```python
from build123d import *

# Parameters (mm, degrees)
CYLINDER002_R     = 2
CYLINDER002_DEPTH = 10
ARRAY002_X_COUNT  = 5
ARRAY002_X_PITCH  = 10
ARRAY002_Y_COUNT  = 3
ARRAY002_Y_PITCH  = 10
CYLINDER001_R     = 1
CYLINDER001_DEPTH = 10
ARRAY001_X_COUNT  = 2
ARRAY001_X_PITCH  = 52
ARRAY001_Y_COUNT  = 2
ARRAY001_Y_PITCH  = 35
BOX_W             = 57
BOX_H             = 40
BOX_DEPTH         = 2


with BuildPart() as array002:
    # Cylinder002 → Cylinder002 (new body)
    with BuildSketch(Plane(origin=(-30, -10, 17), x_dir=(1, 0, 0), z_dir=(0, 0, 1))):
        Circle(CYLINDER002_R)
    extrude(amount=CYLINDER002_DEPTH)

    # Array002 X: Array002 ×5


with BuildPart() as array002_1:
    add(array002.part)
    with Locations(*[(i * ARRAY002_X_PITCH, 0, 0) for i in range(1, ARRAY002_X_COUNT)]):
        add(array002.part)

    # Array002 Y: Array002 ×3


with BuildPart() as array002_2:
    add(array002_1.part)
    with Locations(*[(0, i * ARRAY002_Y_PITCH, 0) for i in range(1, ARRAY002_Y_COUNT)]):
        add(array002_1.part)


with BuildPart() as array001:
    # Cylinder001 → Cylinder001 (new body)
    with BuildSketch(Plane(origin=(-36, -17.5, 18), x_dir=(1, 0, 0), z_dir=(0, 0, 1))):
        Circle(CYLINDER001_R)
    extrude(amount=CYLINDER001_DEPTH)

    # Array001 X: Array001 ×2


with BuildPart() as array001_1:
    add(array001.part)
    with Locations(*[(i * ARRAY001_X_PITCH, 0, 0) for i in range(1, ARRAY001_X_COUNT)]):
        add(array001.part)

    # Array001 Y: Array001 ×2


with BuildPart() as array001_2:
    add(array001_1.part)
    with Locations(*[(0, i * ARRAY001_Y_PITCH, 0) for i in range(1, ARRAY001_Y_COUNT)]):
        add(array001_1.part)


with BuildPart() as top_cut:
    # Box → Box (new body)
    with BuildSketch(Plane(origin=(-38.5, -20, 20.3), x_dir=(1, 0, 0), z_dir=(0, 0, 1))):
        with Locations((28.5, 20)):
            Rectangle(BOX_W, BOX_H)
    extrude(amount=BOX_DEPTH)

    # Cut003: cut Array001
    add(array001_2.part, mode=Mode.SUBTRACT)

    # Cut004: cut Array002
    add(array002_2.part, mode=Mode.SUBTRACT)


solid = top_cut.part
```
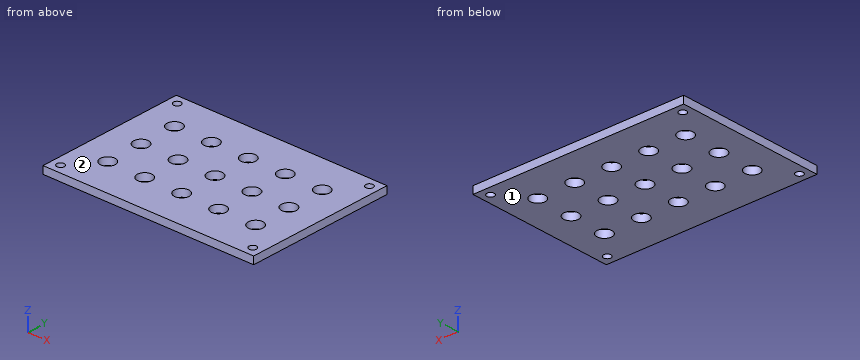
Input: part model. Units: mm. Frame: model coordinates. Face numbers are marked on the shaded views. Round coordinates to 2 decimals unless told otherwise and drop trailing zeros. Loops run counter-clockwise (first coordinate to the right, second up) from the corner with the lowest first, then second, coordinate; pieces in that order, holes last. Notation, with made-up numbers: (63, 58.5) - (68, 58.5) arc R8 ccw to (68, 64.5) - close; hole circle Ø3 at (7.5, 30.25). An arc over 180 degrees is marked (long way). One line per item, written item: value. Start each with the question number.
(1) Section D-D, the plane y = -17.5. Return loops of the section in (x, z), plus the area to 3 significant figures.
(2) Contact query for a flat-ended pin moving along its axis: P1, Ø1.8, axis at x = 16, y = 17.5, coming from the +Z side (3 decimals). Output: stop coordinate, or through.
(3) Draft query along Z for the marked faces 1 and 2. Return one class per face: +Z half, -Z half, draft (parallel to the pull), parting line (faces both ways), or undercut.
(4) Section A-A, the plane x = -30. Return loops of the section in (y, z).
(5) Ray query, line 1 (Y direction, x = -20, z = 21.8); line 2 (X direction, y = 10, z = 21.4); line 3 (Y direction, x = 16, z = 20.8). Return the intervals inside material, ascending. Write a range as [from, to].
(6) Section C-C, the plane z = 21.9. Count the separate pieces of the cut face and the enclosed holes in it, plus the area to 3 significant figures.
(7) Section B-B, the plane y = 0. Return loops of the section in (x, z), plus the area to 3 significant figures.
Results below:
1. outline: (-38.5, 20.3) - (-37, 20.3) - (-37, 22.3) - (-38.5, 22.3) - close; (-35, 20.3) - (15, 20.3) - (15, 22.3) - (-35, 22.3) - close; (17, 20.3) - (18.5, 20.3) - (18.5, 22.3) - (17, 22.3) - close
1. area: 106 mm^2
2. P1: through
3. face 1: -Z half
3. face 2: +Z half
4. outline: (-20, 20.3) - (-12, 20.3) - (-12, 22.3) - (-20, 22.3) - close; (-8, 20.3) - (-2, 20.3) - (-2, 22.3) - (-8, 22.3) - close; (2, 20.3) - (8, 20.3) - (8, 22.3) - (2, 22.3) - close; (12, 20.3) - (20, 20.3) - (20, 22.3) - (12, 22.3) - close
5. line 1: [-20, -12], [-8, -2], [2, 8], [12, 20]
5. line 2: [-38.5, -32], [-28, -22], [-18, -12], [-8, -2], [2, 8], [12, 18.5]
5. line 3: [-20, -18.5], [-16.5, 16.5], [18.5, 20]
6. separate pieces: 1
6. enclosed holes: 19
6. area: 2,080 mm^2
7. outline: (-38.5, 20.3) - (-32, 20.3) - (-32, 22.3) - (-38.5, 22.3) - close; (-28, 20.3) - (-22, 20.3) - (-22, 22.3) - (-28, 22.3) - close; (-18, 20.3) - (-12, 20.3) - (-12, 22.3) - (-18, 22.3) - close; (-8, 20.3) - (-2, 20.3) - (-2, 22.3) - (-8, 22.3) - close; (2, 20.3) - (8, 20.3) - (8, 22.3) - (2, 22.3) - close; (12, 20.3) - (18.5, 20.3) - (18.5, 22.3) - (12, 22.3) - close
7. area: 74.0 mm^2
